For this review, take the finished solid that the model builds, in its own axes (mm). Face numbers are marked on the shaded views. Coordinates: 2 decimals unless noted, no trailing zeros. Order: outer loops, then holes, each group sorted by start corner. A loop starts at its lowest first (then second) coordinate and runs counter-clockwise, first axis right, second up. Notation, with made-up numbers: (-31.5, 0) -> (-25.5, 0) arc R13 ccw to (-25.5, 18) -> close; hole circle Ø9 at (-16, 28.5). An arc over 180 degrees is marked (long way). Return JSON: item names as keys, results as strings. Group by question number.
Item 1: Take a section at D-D (x = -10). Write out the cut boundary in (y, z), then the cut area to 3 significant figures.
Item 2: Take a section at B-B (y = 3). Write out the cut boundary in (x, z).
Item 3: Take a section at A-A (x = -5). Write out the cut boundary in (y, z), then the cut area to 3 significant figures.
Item 4: Draft analysis for pull direction Z (two halves, no side actions). For the marked faces 1, 2 and 3, state which applies: +Z half, -Z half, draft (parallel to the pull), parting line (faces both ways), or undercut.
Item 5: For line 1 along X through (y, z) = (4.25, -7.5); line 2 along Z through (x, y) = (-10, 6); line 3 along X through (y, z) = (5.25, -32.5), list the stretches that pass through material, from the lowest coordinate up.
Item 6: Take a section at C-C (z = -7.5). Write out the cut boundary in (x, y), then the cut area to 3 significant figures.
Autodesk Inventor part; units mm, degrees
ref_plane "YZ Plane" through (0, 0, 0) normal (1, 0, 0) x (0, 1, 0)
ref_plane "XZ Plane" through (0, 0, 0) normal (0, 1, 0) x (-1, 0, 0)
ref_plane "XY Plane" through (0, 0, 0) normal (0, 0, 1) x (1, 0, 0)
sketch "Skizze1" plane through (0, 0, 0) normal (0, 1, 0) x (-1, 0, 0)
  line L0 (0, -48) -> (0, 8)
  line L1 (-10, 0) -> (60, 0)
  line L2 (12.9651, 0) -> (0, 0)
  line L3 (0, 0) -> (0, -40)
  line L4 (0, -40) -> (20, -40)
  line L5 (20, -40) -> (20, -15)
  line L6 (20, -15) -> (50, -15)
  line L7 (50, -15) -> (50, 0)
  line L8 (50, 0) -> (12.9651, 0)
  dimension "d0" = 40
  dimension "d1" = 15
  dimension "d2" = 50
  dimension "d5" = 20
extrude "Extrusion1" add sketch "Skizze1" along normal blind 8
sketch "Skizze2" plane through (0, 8, 0) normal (0, 1, 0) x (1, 0, 0)
  line L0 (-50, 15) -> (-50, 0) construction
  line L1 (-50, 7.5) -> (0, 7.5) construction
  line L2 (0, 0) -> (0, 40) construction
  point P0 (-45, 7.5)
  point P1 (-5, 7.5)
  dimension "d8" = 40
  dimension "d9" = 5
hole "Bohrung1" at (-45, 8, -7.5) at (-5, 8, -7.5) direction (0, -1, 0) diameter 4 end through all
sketch "Skizze3" plane through (0, 8, 0) normal (0, 1, 0) x (1, 0, 0)
  line L0 (0, 40) -> (-20, 40) construction
  line L1 (-10, 40) -> (-10, 0) construction
  line L2 (-50, 0) -> (0, 0) construction
  line L3 (-20, 40) -> (-20, 15) construction
  point P0 (-10, 32.5)
  dimension "d24" = 7.5
hole "Bohrung2" at (-10, 8, -32.5) direction (0, -1, 0) diameter 5.5 end through all
sketch "Skizze4" plane through (0, 8, 0) normal (0, 1, 0) x (1, 0, 0)
  line L0 (0, 40) -> (-20, 40)
  line L1 (-50, 15) -> (-50, 0)
  line L2 (-20, 40) -> (-50, 15)
  line L3 (-50, 15) -> (-20, 15)
  line L4 (-20, 40) -> (-20, 15)
  line L5 (-20, 15) -> (-20, 40)
  point P0 (0, 0)
extrude "Extrusion2" add sketch "Skizze4" against normal up to surface (8 mm away)
fillet "Rundung2" radius 1 2 edges at (0, 4, 0) (-50, 4, 0)
fillet "Rundung3" radius 3 3 edges at (0, 4, -40) (-20, 4, -40) (-50, 4, -15)
properties part number "21_X_Pulley_holder" material "PET-Kunststoff"
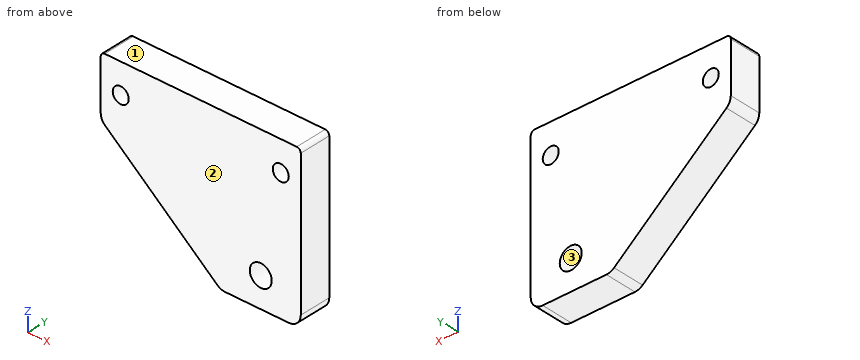
Findings below:
{
 "1": {"outline": "(0, -40) -> (8, -40) -> (8, -35.25) -> (0, -35.25) -> close; (0, -29.75) -> (8, -29.75) -> (8, 0) -> (0, 0) -> close", "area": "276 mm2"},
 "2": {"outline": "(-50, -13.59) arc R3 ccw to (-48.92, -15.9) -> (-20.83, -39.3) arc R3 ccw to (-18.91, -40) -> (-3, -40) arc R3 ccw to (0, -37) -> (0, -1) arc R1 ccw to (-1, 0) -> (-49, 0) arc R1 ccw to (-50, -1) -> close; hole circle Ø4 at (-45, -7.5); hole circle Ø5.5 at (-10, -32.5); hole circle Ø4 at (-5, -7.5)"},
 "3": {"outline": "(0, -40) -> (8, -40) -> (8, -9.5) -> (0, -9.5) -> close; (0, -5.5) -> (8, -5.5) -> (8, 0) -> (0, 0) -> close", "area": "288 mm2"},
 "4": {"face 1": "+Z half", "face 2": "draft", "face 3": "undercut"},
 "5": {"line 1": "x = -50 to -47, -43 to -7, -3 to 0", "line 2": "z = -40 to -35.25, -29.75 to 0", "line 3": "x = -29 to -12.75, -7.25 to 0"},
 "6": {"outline": "(-50, 0) -> (-47, 0) -> (-47, 8) -> (-50, 8) -> close; (-43, 0) -> (-7, 0) -> (-7, 8) -> (-43, 8) -> close; (-3, 0) -> (0, 0) -> (0, 8) -> (-3, 8) -> close", "area": "336 mm2"}
}
